Answer from the drawing. Dimensions are ordinates in mm from the lowest x, y and z of the part. Give positions to 0.01 mm unless a question says otherwise; leave off trailing zeros. Loops run counter-clockwise (first coordinate to the right, second up) from the corner with the lowest first, then second, coordinate; pieces in that order, holes last. Notation, with made-up numbers: (10, 82) - (17, 82) arc R36 ccw to (17, 121) - close; hole circle Ø3 at (39, -9.5). An arc over 180 degrees is marked (long way). Put each result on its own line as item: value. Start each with the question number.
1. Consider L1, parallel to X at y = 0.1, z = 6.5; L2, parallel to X at y = 1.25, z = 7; L3, parallel to Z at x = 20, y = 0.3. Determine where each line is inside the solid, lowest interval first. Write a range as from..to.
2. A cutting plane is placed at D-D, the plane z = 27.5. Determine the outline of the cut face in (x, y).
3. Given pin 1 Ø6 at (x, z) = (35.5, 15.5) entering from -Y, flat-ended and moving along its own axis, determine where the tip first touches the part or whether it passes through.
4. A cutting plane is placed at B-B, the plane x = 21.25. Determine the outline of the cut face in (y, z) (3 decimals).
5. A cutting plane is placed at A-A, the plane z = 6.5. Determine the outline of the cut face in (x, y).
6. A cutting plane is placed at C-C, the plane y = 0.9. Count the separate pieces of the cut face and the enclosed holes in it, plus the area to 3 significant figures.
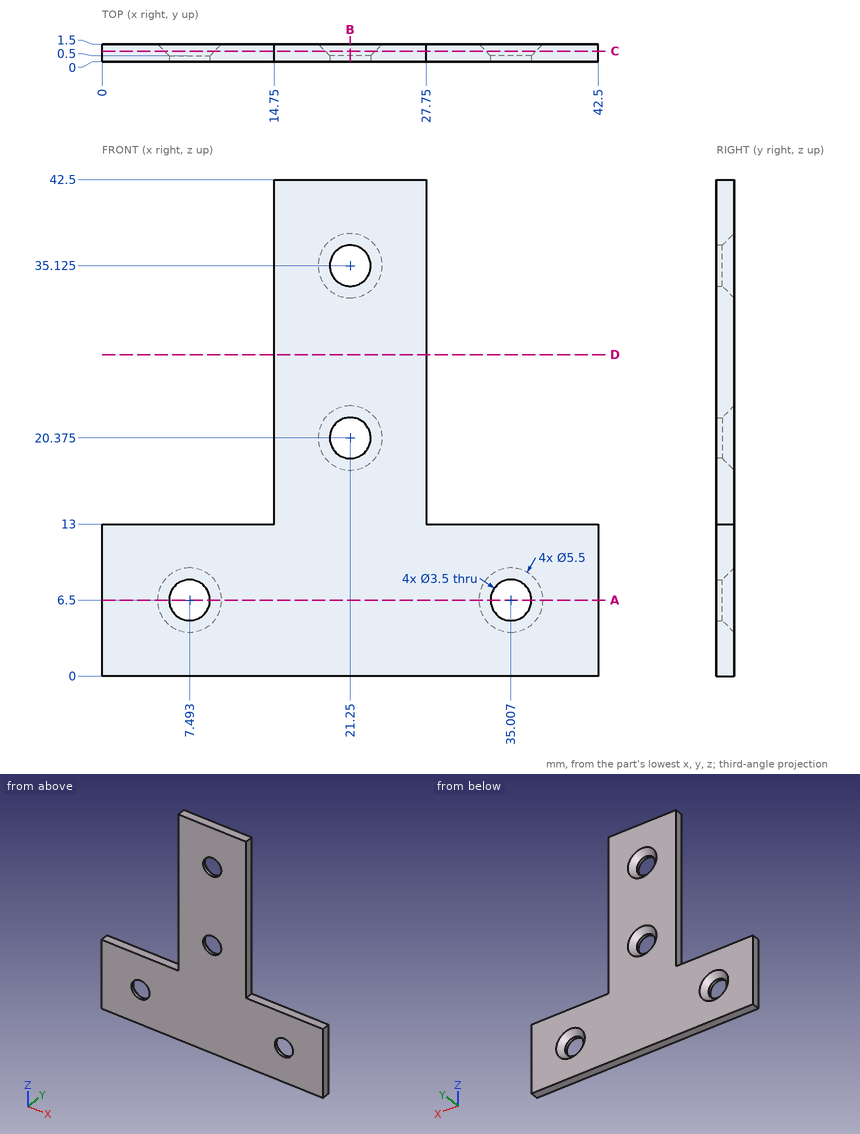
Return value:
1. L1: x = 0..5.74, 9.24..33.26, 36.76..42.5
1. L2: x = 0..5.04, 9.94..32.56, 37.46..42.5
1. L3: z = 0..19.15, 21.6..33.9, 36.35..42.5
2. outline: (14.75, 0) - (27.75, 0) - (27.75, 1.5) - (14.75, 1.5) - close
3. pin 1: stops at y = 0
4. outline: (0, 0) - (1.5, 0) - (1.5, 17.625) - (0.5, 18.625) - (0, 18.625) - close; (0, 22.125) - (0.5, 22.125) - (1.5, 23.125) - (1.5, 32.375) - (0.5, 33.375) - (0, 33.375) - close; (0, 36.875) - (0.5, 36.875) - (1.5, 37.875) - (1.5, 42.5) - (0, 42.5) - close
5. outline: (0, 0) - (5.74, 0) - (5.74, 0.5) - (4.74, 1.5) - (0, 1.5) - close; (9.24, 0) - (33.26, 0) - (33.26, 0.5) - (32.26, 1.5) - (10.24, 1.5) - (9.24, 0.5) - close; (36.76, 0) - (42.5, 0) - (42.5, 1.5) - (37.76, 1.5) - (36.76, 0.5) - close
6. separate pieces: 1
6. enclosed holes: 4
6. area: 878 mm2
